Geometry: final body of the model. Coordinates: model frame, mm. Face numbers are marked on the shaded views. A direction names the side the tool comes from. Round coordinates to 2 decimals unless told otherwise and drop trailing zeros. Loops run counter-clockwise (first coordinate to the right, second up) from the corner with the lowest first, then second, coordinate; pieces in that order, holes last. Notation, with made-up numbers: (31.25, -28) - (90.25, -28) arc R12 cw to (90.25, -18) - close; hole circle Ø2 at (60, 80). An arc over 180 degrees is marked (long way). Write item = value, one per line. Start each with the question number.
Item 1: First-contact query: pin 1 (4 mm diameter, centred on x = 16, y = 30, fed in from -Z); pin 2 (20.5 mm diameter, centred on y = 138.5, z = 64, fed in from -X); pin 3 (8 mm diameter, centred on x = 6.5, z = -16.5, fed in from +Y); pin 4 (8 mm diameter, centred on y = 10, z = -25, fed in from +X). Flat tips, straight axial feed; report the tip coordinate or a pass-through.
Item 2: Section D-D (y = 112.5). Return loops of the section in (x, z), plus the area to 3 significant figures.
Item 3: Access query for the marked faces 1 and 2. Directions: +Z, -Z, +X, -X, +Y, -Y. A direction counts if a zero-diameter tool reaches every point of the face in a straight line with its end or side. Return the directions, or none.
Item 4: Draft query along Z for the marked faces 3, 4, 5 and 6. Return one class per face: pulls with the +Z half, pulls with the -Z half, needs draft (parallel to the pull), parting line crosses it, or undercut.
Item 5: Section A-A (z = -25). Return loops of the section in (x, y), plus the area to 3 significant figures.
Item 6: Line query: line 1 (X direction, y = 18, z = -9); line 2 (Z direction, x = 46, y = 10.5); line 3 (Z direction, x = 41, y = 10). Output: solid intervals per line, ascending. Write a range as from..to.
Item 7: Section C-C (y = 10). Return loops of the section in (x, z), plus the area to 3 significant figures.
from build123d import *

# Parameters (mm, degrees)
BOSS_EXTRUDE1_DEPTH     = 50
SKETCH3_W               = 22
SKETCH3_H               = 20
CUT_EXTRUDE2_DEPTH      = 192.293252092
CUT_EXTRUDE3_DEPTH      = 158.762822921
CUT_EXTRUDE3_DEPTH_BACK = 158.762822921
SKETCH4_R               = 5
FILLET3_R               = 20
CUT_EXTRUDE4_DEPTH      = 162.533613518
CUT_EXTRUDE4_DEPTH_BACK = 162.533613518
SKETCH6_W               = 20
SKETCH6_H               = 30.53527662
BOSS_EXTRUDE2_DEPTH     = 20
SKETCH7_R               = 5
CUT_EXTRUDE5_DEPTH      = 175.536552167
FILLET4_R               = 15.25
FILLET8_R               = 5
CUT_EXTRUDE7_START      = -15
CUT_EXTRUDE7_DEPTH      = 15
CUT_EXTRUDE8_DEPTH      = 15
FILLET13_R              = 1


with BuildPart() as part:
    # Sketch2 → Boss-Extrude1 (new body)
    with BuildSketch(Plane(origin=(0, 0, 0), x_dir=(0, 0, -1), z_dir=(1, 0, 0))):
        with BuildLine():
            Line((0, 0), (50, 0))
            Line((50, 0), (50, 20))
            ThreePointArc((50, 20), (23.281860252, 96.16106544), (-49.46472338, 131.122493479))
            Line((-49.46472338, 131.122493479), (-80, 131.122493479))
            Line((-80, 131.122493479), (-80, 100))
            Line((-80, 100), (-70, 100))
            ThreePointArc((-70, 100), (-18.431457505, 74.497474683), (0, 20))
            Line((0, 20), (0, 0))
        make_face()
    extrude(amount=BOSS_EXTRUDE1_DEPTH)

    # Sketch3 → Cut-Extrude2 (cut, through all)
    with BuildSketch(Plane(origin=(0, 0, -50), x_dir=(-1, 0, 0), z_dir=(0, 0, -1))):
        with Locations((-25, 10)):
            Rectangle(SKETCH3_W, SKETCH3_H)
    extrude(amount=-CUT_EXTRUDE2_DEPTH, mode=Mode.SUBTRACT)

    # Sketch4 → Cut-Extrude3 (cut, two sides: drawn at the far end of the back side and taken through both)
    with BuildSketch(Plane.ZY.offset(-36).offset(-CUT_EXTRUDE3_DEPTH_BACK)):
        with Locations((-25, 10)):
            Circle(SKETCH4_R)
    extrude(amount=CUT_EXTRUDE3_DEPTH + CUT_EXTRUDE3_DEPTH_BACK, mode=Mode.SUBTRACT)

    # Fillet3
    fillet3_edges = [part.edges().sort_by_distance(p)[0] for p in [
        (7, 0, 0),
        (7, 0, -50),
        (43, 0, 0),
        (43, 0, -50),
    ]]
    fillet(fillet3_edges, radius=FILLET3_R - 0.0001)  # a hair under: the kernel refuses the full size

    # Sketch5 → Cut-Extrude4 (cut, two sides: drawn at the far end of the back side and taken through both)
    with BuildSketch(Plane(origin=(0, 0, 0), x_dir=(-1, 0, 0), z_dir=(0, 0, -1)).offset(-CUT_EXTRUDE4_DEPTH_BACK)):
        with BuildLine():
            Line((-36, 20), (-14, 20))
            ThreePointArc((-14, 20), (-25, 31.439818902), (-36, 20))
        make_face()
    extrude(amount=CUT_EXTRUDE4_DEPTH + CUT_EXTRUDE4_DEPTH_BACK, mode=Mode.SUBTRACT)

    # Sketch6 → Boss-Extrude2 (add)
    with BuildSketch(Plane(origin=(0, 131.122493479, 0), x_dir=(1, 0, 0), z_dir=(0, 1, 0))):
        with Locations((25, -64.73236169)):
            Rectangle(SKETCH6_W, SKETCH6_H)
    extrude(amount=BOSS_EXTRUDE2_DEPTH)

    # Sketch7 → Cut-Extrude5 (cut, through all)
    with BuildSketch(Plane(origin=(35, 0, 0), x_dir=(0, 0, -1), z_dir=(1, 0, 0))):
        with Locations((-64.73236169, 141.122493479)):
            Circle(SKETCH7_R)
    extrude(amount=-CUT_EXTRUDE5_DEPTH, mode=Mode.SUBTRACT)

    # Fillet4
    fillet4_edges = [part.edges().sort_by_distance(p)[0] for p in [
        (25, 151.122493479, 80),
        (25, 151.122493479, 49.46472338),
    ]]
    fillet(fillet4_edges, radius=FILLET4_R)

    # Fillet8
    fillet8_edges = [part.edges().sort_by_distance(p)[0] for p in [
        (25, 131.122493479, 49.46472338),
    ]]
    fillet(fillet8_edges, radius=FILLET8_R)

    # Sketch8 → Cut-Extrude7 (cut)
    with BuildSketch(Plane(origin=(50, 0, 0), x_dir=(0, 0, -1), z_dir=(1, 0, 0)).offset(CUT_EXTRUDE7_START)):
        with BuildLine():
            Line((-80, 128.470495387), (-80, 131.122493479))
            Line((-80, 131.122493479), (-49.46472338, 131.122493479))
            ThreePointArc((-49.46472338, 131.122493479), (-47.791514438, 131.016519602), (-46.120201716, 130.883958636))
            ThreePointArc((-46.120201716, 130.883958636), (-62.771967085, 125.632452712), (-80, 128.470495387))
        make_face()
    extrude(amount=CUT_EXTRUDE7_DEPTH, mode=Mode.SUBTRACT)

    # Sketch9 → Cut-Extrude8 (cut)
    with BuildSketch(Plane.ZY):
        with BuildLine():
            Line((80, 128.467222993), (80, 131.122493479))
            Line((80, 131.122493479), (49.46472338, 131.122493479))
            ThreePointArc((49.46472338, 131.122493479), (47.79280742, 131.016611811), (46.122784424, 130.884184126))
            ThreePointArc((46.122784424, 130.884184126), (62.770455841, 125.597808373), (80, 128.467222993))
        make_face()
    extrude(amount=-CUT_EXTRUDE8_DEPTH, mode=Mode.SUBTRACT)

    # Fillet13
    fillet13_edges = [part.edges().sort_by_distance(p)[0] for p in [
        (42.5, 130.883958636, 46.120201716),
        (42.5, 128.470495387, 80),
        (7.5, 128.467222993, 80),
        (7.5, 130.884184126, 46.122784424),
    ]]
    fillet(fillet13_edges, radius=FILLET13_R)


solid = part.part
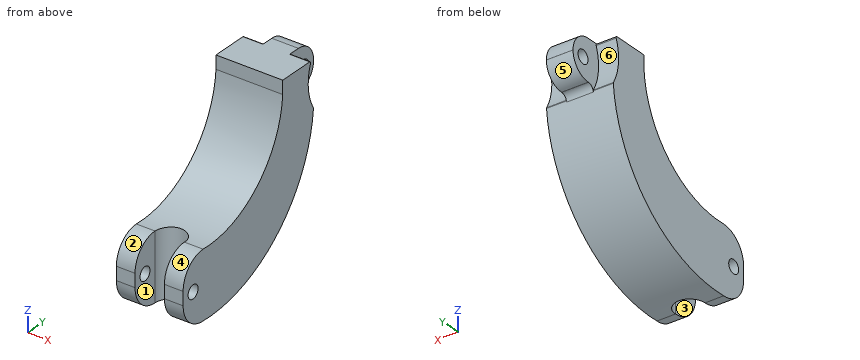
Taken from the geometry:
q1.pin_1 = -50.14
q1.pin_2 = 15
q1.pin_3 = 106.6
q1.pin_4 = through
q2.outline = (0, -4.78) - (50, -4.78) - (50, 80) - (0, 80) - close
q2.area = 4,240 mm^2
q3.face_1 = +Z, -Z, -Y
q3.face_2 = +Z, +X, -X, -Y
q4.face_3 = needs draft
q4.face_4 = pulls with the +Z half
q4.face_5 = pulls with the -Z half
q4.face_6 = undercut
q5.outline = (0, 0) - (14, 0) - (14, 5) - (0, 5) - close; (0, 15) - (14, 15) - (14, 20) arc R11.01 cw (long way) to (36, 20) - (36, 15) - (50, 15) - (50, 94.19) - (0, 94.19) - close; (36, 0) - (50, 0) - (50, 5) - (36, 5) - close
q5.area = 3,790 mm^2
q6.line_1 = 0..14, 36..50
q6.line_2 = -47.6..-29.97, -20.03..-2.4
q6.line_3 = -47.32..-30, -20..-2.68
q7.outline = (0, -47.32) - (14, -47.32) - (14, -30) - (0, -30) - close; (0, -20) - (14, -20) - (14, -2.68) - (0, -2.68) - close; (36, -47.32) - (50, -47.32) - (50, -30) - (36, -30) - close; (36, -20) - (50, -20) - (50, -2.68) - (36, -2.68) - close
q7.area = 970 mm^2
